```python
from build123d import *

# Parameters (mm, degrees)
SKETCH1_R               = 2.0066
SKETCH1_R_2             = 1.2446
BOSS_EXTRUDE1_DEPTH     = 66.675
CUT_EXTRUDE2_DEPTH      = 3.0066
CUT_EXTRUDE2_DEPTH_BACK = 3.0066
CUT_EXTRUDE3_DEPTH      = 3.0066
CUT_EXTRUDE3_DEPTH_BACK = 3.0066


with BuildPart() as part:
    # Sketch1 → Boss-Extrude1 (new body)
    with BuildSketch(Plane(origin=(0, 0, 0), x_dir=(0, 0, -1), z_dir=(1, 0, 0))):
        Circle(SKETCH1_R)
        Circle(SKETCH1_R_2, mode=Mode.SUBTRACT)
    extrude(amount=BOSS_EXTRUDE1_DEPTH)

    # Sketch3 → Cut-Extrude2 (cut, two sides)
    with BuildSketch(Plane.XY) as cut_extrude2_sk:
        Polygon((0, 2.0066), (2.0066, 0), (0, -2.0066), align=None)
    extrude(amount=CUT_EXTRUDE2_DEPTH, mode=Mode.SUBTRACT)
    extrude(cut_extrude2_sk.sketch, amount=-CUT_EXTRUDE2_DEPTH_BACK, mode=Mode.SUBTRACT)

    # Sketch4 → Cut-Extrude3 (cut, two sides)
    with BuildSketch(Plane(origin=(0, 0, 0), x_dir=(1, 0, 0), z_dir=(0, 1, 0))) as cut_extrude3_sk:
        Polygon((66.675, 2.0066), (64.6684, 0), (66.675, -2.0066), align=None)
    extrude(amount=CUT_EXTRUDE3_DEPTH, mode=Mode.SUBTRACT)
    extrude(cut_extrude3_sk.sketch, amount=-CUT_EXTRUDE3_DEPTH_BACK, mode=Mode.SUBTRACT)


solid = part.part
```
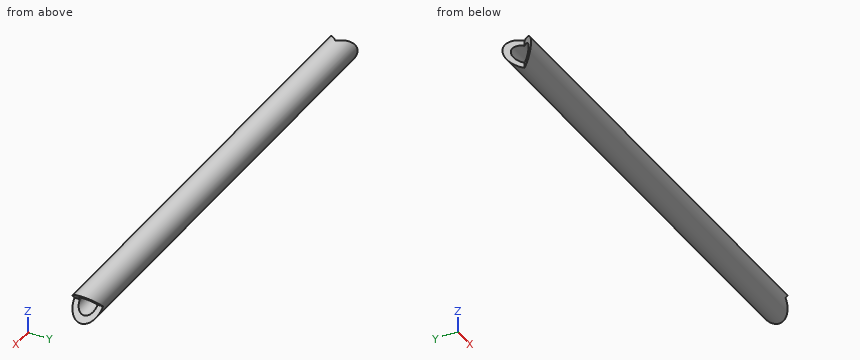
Work out the finished part from the listing and answer in its coordinate system (mm). Round coordinates to 2 decimals unless told otherwise and drop trailing zeros. Write each loop counter-clockwise with the first axis right and the second up, starting at its lowest first coordinate (ties: lowest second). Pieces come first, ordered by that corner, then holes. Notation, with made-up numbers: (-10, 44.25) - (-4, 44.25) arc R37 ccw to (-4, 81.25) - close; hole circle Ø7 at (-4.5, -28). An arc over 180 degrees is marked (long way). Return JSON: item names as keys, results as strings. Group by question number.
Q1. The part is cut by section A-A on y = 0.7. Write down the section's boundary in (x, z).
Q2. This flat-tipped pin is pushed along its axis until it touches: pin 1 Ø1.5 at (x, y) = (36, 1.5) entering from +Z. Where does it stop, or does it pass through?
Q3. Find the intervals of material crossed by L1, parallel to Y at x = 40, z = 0; L2, parallel to Y at x = 27.5, z = 0.55, in increasing order.
Q4. The part is cut by section B-B on x = 56. Write down the section's boundary in (y, z).
Solved:
{
 "1": {"outline": "(1.31, -1.88) - (66.55, -1.88) - (65.7, -1.03) - (1.31, -1.03) - close; (1.31, 1.03) - (65.7, 1.03) - (66.55, 1.88) - (1.31, 1.88) - close"},
 "2": {"pin 1": "z = 1.86"},
 "3": {"L1": "-2.01 to -1.24, 1.24 to 2.01", "L2": "-1.93 to -1.12, 1.12 to 1.93"},
 "4": {"outline": "circle Ø4.01 at (0, 0); hole circle Ø2.49 at (0, 0)"}
}
